```python
from build123d import *

# Parameters (mm, degrees)
SKETCH1_W               = 100
SKETCH1_H               = 100
BOSS_EXTRUDE1_DEPTH     = 4
SKETCH2_R               = 4.25
BOSS_EXTRUDE2_DEPTH     = 30
SKETCH4_R               = 4.75
CUT_EXTRUDE1_DEPTH      = 1.5
SKETCH5_R               = 2
SKETCH5_R_2             = 5
CUT_EXTRUDE2_DEPTH      = 31
CUT_EXTRUDE2_DEPTH_BACK = 5
SKETCH6_W               = 20
SKETCH6_H               = 10
SKETCH6_R               = 1.75
BOSS_EXTRUDE3_DEPTH     = 8
SKETCH7_R               = 5.5
CUT_EXTRUDE3_DEPTH      = 8


with BuildPart() as part:
    # Sketch1 → Boss-Extrude1 (new body)
    with BuildSketch(Plane.XY):
        Rectangle(SKETCH1_W, SKETCH1_H)
    extrude(amount=BOSS_EXTRUDE1_DEPTH)

    # Sketch2 → Boss-Extrude2 (add)
    with BuildSketch(Plane.XY.offset(4)):
        with Locations((45, 45)):
            Circle(SKETCH2_R)
        with Locations((-45, 45)):
            Circle(SKETCH2_R)
        with Locations((-45, -45)):
            Circle(SKETCH2_R)
        with Locations((45, -45)):
            Circle(SKETCH2_R)
    extrude(amount=BOSS_EXTRUDE2_DEPTH)

    # Sketch4 → Cut-Extrude1 (cut)
    with BuildSketch(Plane(origin=(0, 0, 0), x_dir=(-1, 0, 0), z_dir=(0, 0, -1))):
        with Locations((-45, 45)):
            Circle(SKETCH4_R)
        with Locations((45, 45)):
            Circle(SKETCH4_R)
        with Locations((-45, -45)):
            Circle(SKETCH4_R)
        with Locations((45, -45)):
            Circle(SKETCH4_R)
    extrude(amount=-CUT_EXTRUDE1_DEPTH, mode=Mode.SUBTRACT)

    # Sketch5 → Cut-Extrude2 (cut, two sides)
    with BuildSketch(Plane(origin=(-38.404344239, -79.614153906, 4), x_dir=(1, 0, 0), z_dir=(0, 0, 1))) as cut_extrude2_sk:
        with Locations((36.292632212, 51.750208167)):
            Circle(SKETCH5_R)
        with Locations((1.292632212, 51.750208167)):
            Circle(SKETCH5_R)
        with Locations((18.792632212, 59.750208167)):
            Circle(SKETCH5_R_2)
    extrude(amount=CUT_EXTRUDE2_DEPTH, mode=Mode.SUBTRACT)
    extrude(cut_extrude2_sk.sketch, amount=-CUT_EXTRUDE2_DEPTH_BACK, mode=Mode.SUBTRACT)

    # Sketch6 → Boss-Extrude3 (add)
    with BuildSketch(Plane.XY.offset(4)):
        with Locations((-25.571153041, 19.73100851)):
            Rectangle(SKETCH6_W, SKETCH6_H)
        with Locations((-32.571153041, 19.73100851)):
            Circle(SKETCH6_R, mode=Mode.SUBTRACT)
    extrude(amount=BOSS_EXTRUDE3_DEPTH)

    # Sketch7 → Cut-Extrude3 (cut)
    with BuildSketch(Plane(origin=(-38.404344239, -79.614153906, 0), x_dir=(-1, 0, 0), z_dir=(0, 0, -1))):
        with Locations((-58.387586461, 99.345162416)):
            Circle(SKETCH7_R)
    extrude(amount=-CUT_EXTRUDE3_DEPTH, mode=Mode.SUBTRACT)


solid = part.part
```
The model under review builds one solid part; all positions refer to its coordinate system, in mm. A direction names the side the tool comes from. Round coordinates to 2 decimals unless told otherwise and drop trailing zeros. Write each loop counter-clockwise with the first axis right and the second up, starting at its lowest first coordinate (ties: lowest second). Pieces come first, ordered by that corner, then holes. Notation, with made-up numbers: (-39.75, 84) - (13.25, 84) arc R20 ccw to (13.25, 121) - close; hole circle Ø2 at (23.5, 78.5). An arc over 180 degrees is marked (long way). One line per question, with ' | ' between items.
Item 1: The part is to be moulded in two halves that separate along Y. For faces 1 (the face through (-26, 14.731, 8)), 2 (the face through (-31.63, 21.207, 7.944)), 3 (the face through (-26, 20, 12)), say which applies: pulls with the +Y half, pulls with the -Y half, needs draft (parallel to the pull), parting line crosses it, or undercut.
Resolved:
face 1: pulls with the -Y half | face 2: undercut | face 3: needs draft
Item 2: Add section B-B, the plane x = -45. Give the boundary of the cut face in (y, z).
Resolved:
outline: (-50, 0) - (-49.75, 0) - (-49.75, 1.5) - (-40.25, 1.5) - (-40.25, 0) - (40.25, 0) - (40.25, 1.5) - (49.75, 1.5) - (49.75, 0) - (50, 0) - (50, 4) - (49.25, 4) - (49.25, 34) - (40.75, 34) - (40.75, 4) - (-40.75, 4) - (-40.75, 34) - (-49.25, 34) - (-49.25, 4) - (-50, 4) - close
Item 3: Add section D-D, the plane z = 17. Give the boundary of the cut face in (x, y), then the cut area to 3 significant figures.
Resolved:
outline: circle Ø8.5 at (-45, -45); circle Ø8.5 at (-45, 45); circle Ø8.5 at (45, -45); circle Ø8.5 at (45, 45) | area: 227 mm2
Item 4: To check wall thickness, follow probe 1 along Y at (x, z) = (-45, 1); probe 2 along X at (y, z) = (-27.5, 3); probe 3 along Z at (x, y) = (-25, 46.5). State the ranges of each line that lie inside material, in increasing order.
Resolved:
probe 1: y = -50 to -49.75, -40.25 to 40.25, 49.75 to 50 | probe 2: x = -50 to -39.08, -35.15 to -4.08, -0.15 to 50 | probe 3: z = 0 to 4
Item 5: Add section A-A, the plane z = 9. Give the boundary of the cut face in (x, y).
Resolved:
outline: circle Ø8.5 at (-45, -45); circle Ø8.5 at (-45, 45); (-35.57, 14.73) - (-15.57, 14.73) - (-15.57, 24.73) - (-35.57, 24.73) - close; circle Ø8.5 at (45, -45); circle Ø8.5 at (45, 45); hole circle Ø3.5 at (-32.57, 19.73)
Item 6: For faces 4 (the face through (45, 45, 1.5)), 5 (the face through (-15.571, 20, 8)), 6 (the face through (-24.607, -19.644, 2.028)), 7 (the face through (41.63, 42.41, 18.79)), list the 3-axis set-ups (+Z, -Z, +X, -X, +Y, -Y) from which the entire face can be reached by the end or side of a thin tool; tool diameter is ignored.
Resolved:
face 4: -Z | face 5: +Z, +X, +Y, -Y | face 6: +Z, -Z | face 7: +Z
Item 7: For P1, Ø3.5, axis at x = -37.11, y = -27.86, coming from the +Z side; P2, Ø12, axis at x = -3.5, y = -7, coming from the +Z side; P3, Ø2.5, axis at y = 21.5, z = 6.5, coming from the +X side; P4, Ø3, axis at x = -21, y = 21, coming from the +Z side, all flat-tipped, find the tip position at first contact; note any pin that passes through.
Resolved:
P1: passes through | P2: stops at z = 4 | P3: stops at x = -15.57 | P4: stops at z = 12
